Autodesk Inventor part; units mm, degrees
ref_plane "YZ Plane" through (0, 0, 0) normal (1, 0, 0) x (0, 1, 0)
ref_plane "XZ Plane" through (0, 0, 0) normal (0, 1, 0) x (-1, 0, 0)
ref_plane "XY Plane" through (0, 0, 0) normal (0, 0, 1) x (1, 0, 0)
sketch "Sketch1" plane through (0, 0, 0) normal (0, 1, 0) x (-1, 0, 0)
  line L0 (-5.1, 9.9) -> (5.1, 9.9)
  line L1 (5.1, 9.9) -> (5.1, 0.75)
  line L2 (5.1, -9.9) -> (4.4, -9.9) construction
  line L3 (-5.1, -9.9) -> (-5.1, 9.9)
  line L4 (-5.1, 9.9) -> (5.1, -9.9) construction
  line L5 (5.1, 9.9) -> (-5.1, -9.9) construction
  line L6 (0, 9.9) -> (0, 4.8) construction
  line L7 (0, 9.9) -> (5.1, 9.9) construction
  line L8 (-5.1, 4.8) -> (-2.6, 4.8) construction
  circle A0 centre (-2.6, 4.8) radius 1.25
  line L9 (-2.6, 4.8) -> (-2.6, -4.7) construction
  line L10 (-2.6, 4.8) -> (6.9, 4.8) construction
  circle A1 centre (-2.6, -4.7) radius 1.25
  line L11 (-5.1, -9.9) -> (4.4, -9.9) construction
  line L12 (-5.1, -9.9) -> (4.4, -9.9) construction
  line L13 (4.4, -9.9) -> (4.4, 0.05)
  line L14 (4.4, 0.05) -> (5.1, 0.75)
  line L15 (5.1, 0.75) -> (5.1, -9.9) construction
  line L16 (4.4, -9.9) -> (-5.1, -9.9)
  point P0 (0, 0)
  dimension "d0" = 10.2
  dimension "d1" = 19.8
  dimension "d3" = 90
  dimension "d4" = 2.5
  dimension "d5" = 5.1
  dimension "d6" = 0
  dimension "d7" = 2.5
  dimension "d8" = 9.5
  dimension "d9" = 90
  dimension "d10" = 2.5
  dimension "d11" = 9.5
  dimension "d12" = 0
  dimension "d13" = 135
  dimension "d14" = 3.0759
extrude "Extrusion1" add sketch "Sketch1" along normal mid plane 6.4
sketch "Sketch2" plane through (0, 0, 0) normal (0, 1, 0) x (-1, 0, 0)
  line L0 (5.1, 9.9) -> (-5.1, 9.9) construction
  line L1 (-5.1, -9.9) -> (5.1, -9.9) construction
  line L2 (5.1, -9.9) -> (5.1, 9.9) construction
  line L3 (5.1, 9.9) -> (-5.1, 9.9) construction
  line L4 (-5.1, 9.9) -> (-5.1, -9.9) construction
  line L5 (-5.1, -9.9) -> (5.1, 9.9) construction
  line L6 (5.1, -9.9) -> (-5.1, 9.9) construction
  line L7 (5.1, 9.9) -> (5.1, 7.1) construction
  line L8 (5.1, 0.75) -> (5.1, 9.9)
  line L9 (5.1, 9.9) -> (7.9, 9.9) construction
  line L10 (5.1, 7.1) -> (7, 7.1) construction
  line L11 (5.1, 7.1) -> (7, 7.1) construction
  line L12 (7, 7.1) -> (7, -9.9) construction
  line L13 (6, 8.1) -> (8, 8.1) construction
  line L14 (8, 8.1) -> (8, 6.1) construction
  line L15 (8, 6.1) -> (6, 6.1) construction
  line L16 (6, 6.1) -> (6, 8.1) construction
  line L17 (6, 8.1) -> (8, 6.1) construction
  line L18 (8, 8.1) -> (6, 6.1) construction
  line L19 (5.1, 7.1) -> (6, 7.1)
  arc A0 (7, 6.1) -> (6, 7.1) centre (6, 6.1) ccw
  line L20 (7, 6.1) -> (7, -9.9)
  line L21 (7, -9.9) -> (6.8, -9.9)
  line L22 (6.8, -9.9) -> (6.8, 6.1)
  line L23 (5.1, 7.1) -> (5.1, 6.9)
  line L24 (5.1, 6.9) -> (6, 6.9)
  arc A1 (6.8, 6.1) -> (6, 6.9) centre (6, 6.1) ccw
  point P0 (0, 0)
  dimension "d17" = 2.8
  dimension "d18" = 90
  dimension "d19" = 1.9
  dimension "d20" = 0
  dimension "d21" = 2
  dimension "d22" = 2
  dimension "d23" = 0.2
  dimension "d24" = 90
  dimension "d25" = 0.2
extrude "Extrusion2" add sketch "Sketch2" along normal mid plane 3.8
sketch "Sketch3" plane through (0, 0, 0) normal (0, 1, 0) x (-1, 0, 0)
  line L0 (-5.1, 9.9) -> (-5.1, -9.9) construction
  line L1 (5.1, 9.9) -> (-5.1, 9.9) construction
  line L2 (-5.1, 9.9) -> (-5.1, -9.9) construction
  line L3 (-5.1, -9.9) -> (5.1, -9.9) construction
  line L4 (5.1, -9.9) -> (5.1, 9.9) construction
  line L5 (5.1, 9.9) -> (-5.1, -9.9) construction
  line L6 (-5.1, 9.9) -> (5.1, -9.9) construction
  line L7 (-5.1, 9.9) -> (-5.1, 7.9) construction
  line L8 (-5.1, 7.9) -> (-5.1, -0.9) construction
  line L9 (-5.1, -0.9) -> (-5.1, -8.2) construction
  line L10 (-9.1, 8.15) -> (-1.1, 8.15)
  line L11 (-1.1, 8.15) -> (-1.1, 7.65)
  line L12 (-1.1, 7.65) -> (-9.1, 7.65)
  line L13 (-9.1, 7.65) -> (-9.1, 8.15)
  line L14 (-9.1, 8.15) -> (-1.1, 7.65) construction
  line L15 (-1.1, 8.15) -> (-9.1, 7.65) construction
  line L16 (-9.1, -0.65) -> (-1.1, -0.65)
  line L17 (-1.1, -0.65) -> (-1.1, -1.15)
  line L18 (-1.1, -1.15) -> (-9.1, -1.15)
  line L19 (-9.1, -1.15) -> (-9.1, -0.65)
  line L20 (-9.1, -0.65) -> (-1.1, -1.15) construction
  line L21 (-1.1, -0.65) -> (-9.1, -1.15) construction
  line L22 (-9.1, -8.45) -> (-1.1, -8.45)
  line L23 (-1.1, -8.45) -> (-1.1, -7.95)
  line L24 (-1.1, -7.95) -> (-9.1, -7.95)
  line L25 (-9.1, -7.95) -> (-9.1, -8.45)
  line L26 (-9.1, -8.45) -> (-1.1, -7.95) construction
  line L27 (-1.1, -8.45) -> (-9.1, -7.95) construction
  point P0 (0, 0)
  dimension "d28" = 2
  dimension "d29" = 8.8
  dimension "d30" = 7.3
  dimension "d31" = 8
  dimension "d32" = 0.5
  dimension "d33" = 8
  dimension "d34" = 0.5
  dimension "d35" = 8
  dimension "d36" = 0.5
extrude "Extrusion3" add sketch "Sketch3" along normal mid plane 3.2
sketch "Sketch4" plane through (5.1, -1.6, 8.15) normal (0, 0, 1) x (1, 0, 0)
  line L0 (0, 3.2) -> (4, 3.2) construction
  line L1 (4, 0) -> (0, 0) construction
  line L2 (4, 3.2) -> (0.8, 3.2) construction
  line L3 (0.8, 3.2) -> (0.8, 0) construction
  line L4 (0.8, 0) -> (4, 0) construction
  line L5 (4, 0) -> (4, 3.2) construction
  line L6 (0.8, 3.2) -> (4, 0) construction
  line L7 (0.8, 0) -> (4, 3.2) construction
  circle A0 centre (2.4, 1.6) radius 0.8
  point P0 (-5.1, 1.6)
  dimension "d39" = 3.2
  dimension "d40" = 1.6
extrude "Extrusion4" cut sketch "Sketch4" against normal blind 40
fillet "Fillet1" radius 1 6 edges at (5.1, 0, 9.9) (-5.1, 0, 9.9) (-4.4, 0, -9.9) (5.1, 0, -9.9) (-4.4, 0, 0.05) (-5.1, 0, 0.75)
fillet "Fillet2" radius 0.5 6 edges at (9.1, 1.6, -8.2) (9.1, -1.6, -8.2) (9.1, -1.6, -0.9) (9.1, 1.6, -0.9) (9.1, -1.6, 7.9) (9.1, 1.6, 7.9)
properties part number "endstop_maszyna"
Source: CAD feature listing. Evaluate the final solid. Frame: model axes, mm. A direction names the side the tool comes from. Coordinates: 2 decimals unless noted, no trailing zeros. Loops run counter-clockwise (first coordinate to the right, second up) from the corner with the lowest first, then second, coordinate; pieces in that order, holes last. Notation, with made-up numbers: M 70.25,76 L 85.25,76 A34 cw 85.25,110 Z; hole C 60.25,89 d4. An arc over 180 degrees is marked long. Use a Markdown table: item, result. Add a question column.
Q1. Material intervals for L1, parallel to Z at x = 6, y = -1; L2, parallel to Z at x = 2.6, y = -1.25; L3, parallel to X at y = 0.5, z = -3.25, sorted ascending.
Q2. Section query A-A, the plane x = 7.5. Return loops of the section in (y, z), and give its area (3 significant figures).
Q3. Draft query along Z for faces 6 (the flat face through (5.1, 0, 0)), 7 (the flat face through (0, 0, -9.9)), 8 (the flat face through (0, 3.2, 0)). Return one class per face: pulls with the +Z half, pulls with the -Z half, needs draft (parallel to the pull), parting line crosses it, or undercut.
Q4. Section query B-B, the plane z = 2.5. Return loops of the section in (x, y), and give its area (3 significant figures).
Q5. Section query C-C, the plane x = 2.6. Return loops of the section in (y, z), and give its area (3 significant figures).
Q6. Section query D-D, the plane z = 4.8. Return loops of the section in (x, y), and give its area (3 significant figures).
Q7. Access query for faces 1 (the flat face through (-5.5, 0, 7.1)), 2 (the flat face through (6.6, -0.4, -7.95)), 3 (the cylindrical face through (-4.099, 0.045, -9.615)), 4 (the flat face through (7, -1, -8.45)), 5 (the cylindrical face through (1.928, -0.045, 3.746)). Directions: +Z, -Z, +X, -X, +Y, -Y. A direction counts if a zero-diameter tool reaches every point of the face in a straight line with its end or side. Return the directions, or none.
Q8. First-contact query: pin 1 (2.5 mm diameter, centred on x = 8, y = 0, fed in from -Z); pin 2 (1.4 mm diameter, centred on x = 7.5, y = 0, fed in from +Z); pin 3 (1.5 mm diameter, centred on y = 2, z = -1.5, fed in from +X); pin 4 (0.7 mm diameter, centred on x = -5.5, y = 0.5, fed in from -Z). Flat tips, straight axial feed; report the tip coordinate or a pass-through.
Result:
| question | item | result |
|---|---|---|
| 1 | L1 | z = -8.45 to -7.95, -1.15 to -0.65, 7.65 to 8.15 |
| 1 | L2 | z = -9.9 to -5.95, -3.45 to 3.55, 6.05 to 9.9 |
| 1 | L3 | x = -7 to -6.8, -4.4 to 5.1 |
| 2 | outline | M -1.6,-8.45 L -0.8,-8.45 L -0.8,-7.95 L -1.6,-7.95 Z; M -1.6,-1.15 L -0.8,-1.15 L -0.8,-0.65 L -1.6,-0.65 Z; M -1.6,7.65 L -0.8,7.65 L -0.8,8.15 L -1.6,8.15 Z; M 0.8,-8.45 L 1.6,-8.45 L 1.6,-7.95 L 0.8,-7.95 Z; M 0.8,-1.15 L 1.6,-1.15 L 1.6,-0.65 L 0.8,-0.65 Z; M 0.8,7.65 L 1.6,7.65 L 1.6,8.15 L 0.8,8.15 Z |
| 2 | area | 2.40 mm2 |
| 3 | face 6 | undercut |
| 3 | face 7 | pulls with the -Z half |
| 3 | face 8 | needs draft |
| 4 | outline | M -7,-1.9 L -6.8,-1.9 L -6.8,1.9 L -7,1.9 Z; M -5.1,-3.2 L 5.1,-3.2 L 5.1,3.2 L -5.1,3.2 Z |
| 4 | area | 66.0 mm2 |
| 5 | outline | M -3.2,-9.9 L 3.2,-9.9 L 3.2,-5.95 L -3.2,-5.95 Z; M -3.2,-3.45 L 3.2,-3.45 L 3.2,3.55 L -3.2,3.55 Z; M -3.2,6.05 L 3.2,6.05 L 3.2,9.9 L -3.2,9.9 Z |
| 5 | area | 94.7 mm2 |
| 6 | outline | M -7,-1.9 L -6.8,-1.9 L -6.8,1.9 L -7,1.9 Z; M -5.1,-3.2 L 1.35,-3.2 L 1.35,3.2 L -5.1,3.2 Z; M 3.85,-3.2 L 5.1,-3.2 L 5.1,3.2 L 3.85,3.2 Z |
| 6 | area | 50.0 mm2 |
| 7 | face 1 | +Z, -X, +Y, -Y |
| 7 | face 2 | +X, +Y, -Y |
| 7 | face 3 | -Z, +Y, -Y |
| 7 | face 4 | -Z, +X, +Y, -Y |
| 7 | face 5 | +Y, -Y |
| 8 | pin 1 | stops at z = -8.45 |
| 8 | pin 2 | passes through |
| 8 | pin 3 | stops at x = 9.04 |
| 8 | pin 4 | stops at z = 6.9 |
